```python
from build123d import *

# Parameters (mm, degrees)
F0_R     = 17.78
F1_DEPTH = 2.54
F2_R     = 17.78
F2_R_2   = 16.51
F3_DEPTH = 1.27
F4_R     = 17.78
F5_DEPTH = 2.54
F6_R     = 14.605
F7_DEPTH = 50.8
F8_R     = 2.54


with BuildPart() as f1:
    # F0 (on Top) → F1 (new body)
    with BuildSketch(Plane.XY):
        Circle(F0_R)
    extrude(amount=F1_DEPTH)

    # F2 (on face) → F3 (join)
    with BuildSketch(Plane.XY.offset(2.54)):
        Circle(F2_R)
        Circle(F2_R_2, mode=Mode.SUBTRACT)
    extrude(amount=F3_DEPTH)

    # F4 (on face) → F5 (join)
    with BuildSketch(Plane.XY.offset(3.81)):
        Circle(F4_R)
    extrude(amount=F5_DEPTH)

    # F6 (on face) → F7 (cut)
    with BuildSketch(Plane(origin=(0, 0, 0), x_dir=(1, 0, 0), z_dir=(0, 0, -1))):
        Circle(F6_R)
    extrude(amount=-F7_DEPTH, mode=Mode.SUBTRACT)

    # F8
    f8_edges = [f1.edges().sort_by_distance(p)[0] for p in [
        (-17.78, 0, 6.35),
        (-17.78, 0, 0),
    ]]
    fillet(f8_edges, radius=F8_R)


solid = f1.part
```
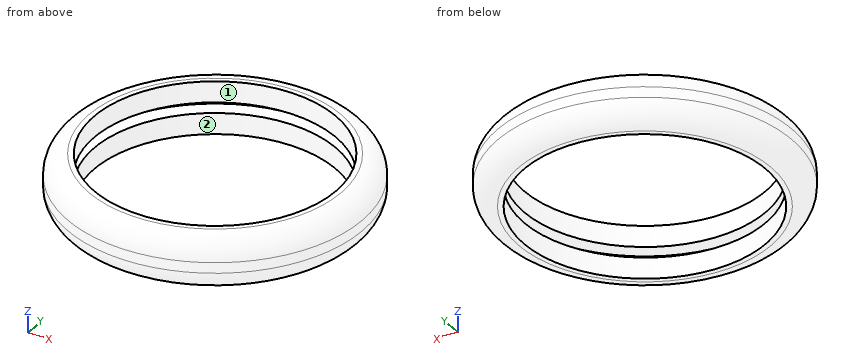
Here's how the part is built. I have some questions about the finished solid (model axes, mm). Face numbers are marked on the shaded views. Give positions to 0.01 mm unless a question says otherwise; leave off trailing zeros. Loops run counter-clockwise (first coordinate to the right, second up) from the corner with the lowest first, then second, coordinate; pieces in that order, holes last. Notation, with made-up numbers: M -30.75,49 L -14.75,49 A12 ccw -14.75,56 Z; hole C 28,-8.75 d6. An arc over 180 degrees is marked long. Put each result on its own line as item: value. Start each with the question number.
(1) I need wall thicknesses on line 1 along Y through (x, z) = (0.5, 3.75); line 2 along Z through (x, y) = (-4.5, 14); line 3 along X through (y, z) = (-2, 4.25). Which ranges of each line are inside material? Lowest first, please. Write a range as [from, to].
(2) Will these pins go through, and if not, where does the flat tip stop? pin 1 Ø10 at (x, y) = (9, 11) entering from +Z; pin 2 Ø6 at (x, y) = (4, -8) entering from -Z; pin 3 Ø2 at (x, z) = (6.5, 2.5) entering from -Y; pin 4 Ø3 at (y, z) = (4, 2.5) entering from -X.
(3) If we mould it in two halves opening along X, with no side actions, what happens to the marked faces 1 and 2? For each: +X half, -X half, draft (parallel to the pull), parting line (faces both ways), or undercut.
(4) I want a section at A-A on x = 0. Please give me the cut outline in (y, z) (3 decimals).
(5) I want a section at C-C on z = 5. Please give me the cut outline in (x, y) (3 decimals).
Answer block:
1. line 1: [-17.77, -16.5], [16.5, 17.77]
1. line 2: [0, 2.54], [3.81, 6.35]
1. line 3: [-17.63, -14.47], [14.47, 17.63]
2. pin 1: z = 6.35
2. pin 2: through
2. pin 3: y = -16.91
2. pin 4: x = -17.6
3. face 1: undercut
3. face 2: undercut
4. outline: M -17.78,2.54 A2.54 ccw -15.24,0 L -14.605,0 L -14.605,2.54 L -16.51,2.54 L -16.51,3.81 L -14.605,3.81 L -14.605,6.35 L -15.24,6.35 A2.54 ccw -17.78,3.81 Z; M 14.605,0 L 15.24,0 A2.54 ccw 17.78,2.54 L 17.78,3.81 A2.54 ccw 15.24,6.35 L 14.605,6.35 L 14.605,3.81 L 16.51,3.81 L 16.51,2.54 L 14.605,2.54 Z
5. outline: C 0,0 d34.968; hole C 0,0 d29.21
